```python
from build123d import *

# Parameters (mm, degrees)
SKETCH1_W           = 11.8
SKETCH1_H           = 22.5
BOSS_EXTRUDE1_DEPTH = 23.3
SKETCH2_W           = 11.8
SKETCH2_H           = 31.9
SKETCH2_R           = 1
BOSS_EXTRUDE2_DEPTH = 2.5
SKETCH3_R           = 5.9
SKETCH3_R_2         = 2.5
BOSS_EXTRUDE3_DEPTH = 4
SKETCH4_R           = 2.3
BOSS_EXTRUDE4_DEPTH = 3.2
SKETCH5_W           = 3.6
SKETCH5_H           = 1.2
BOSS_EXTRUDE5_DEPTH = 8


with BuildPart() as part:
    # Sketch1 → Boss-Extrude1 (new body)
    with BuildSketch(Plane(origin=(0, 0, 0), x_dir=(1, 0, 0), z_dir=(0, 1, 0))):
        Rectangle(SKETCH1_W, SKETCH1_H)
    extrude(amount=BOSS_EXTRUDE1_DEPTH)

    # Sketch2 → Boss-Extrude2 (add)
    with BuildSketch(Plane(origin=(0, 16.6, 0), x_dir=(1, 0, 0), z_dir=(0, 1, 0))):
        Rectangle(SKETCH2_W, SKETCH2_H)
        with Locations(Location((0, 13.65, 0), (0, 0, 270))):
            Circle(SKETCH2_R, mode=Mode.SUBTRACT)
        with Locations(Location((0, -13.65, 0), (0, 0, 90))):
            Circle(SKETCH2_R, mode=Mode.SUBTRACT)
    extrude(amount=BOSS_EXTRUDE2_DEPTH)

    # Sketch3 → Boss-Extrude3 (add)
    with BuildSketch(Plane(origin=(0, 23.3, 0), x_dir=(1, 0, 0), z_dir=(0, 1, 0))):
        with Locations((0, -5.35)):
            Circle(SKETCH3_R)
        with Locations((0, 0.95)):
            Circle(SKETCH3_R_2)
    extrude(amount=BOSS_EXTRUDE3_DEPTH)

    # Sketch4 → Boss-Extrude4 (add)
    with BuildSketch(Plane(origin=(0, 27.3, 0), x_dir=(1, 0, 0), z_dir=(0, 1, 0))):
        with Locations(Location((0, -5.35, 0), (0, 0, 270))):
            Circle(SKETCH4_R)
    extrude(amount=BOSS_EXTRUDE4_DEPTH)

    # Sketch5 → Boss-Extrude5 (add)
    with BuildSketch(Plane.XY.offset(11.25)):
        with Locations((0, 5.1)):
            Rectangle(SKETCH5_W, SKETCH5_H)
    extrude(amount=BOSS_EXTRUDE5_DEPTH)


solid = part.part
```
Check sheet for the modelled part. Datum: model origin and axes. Units: mm. A direction names the side the tool comes from. Round coordinates to 2 decimals unless told otherwise and drop trailing zeros. Loops run counter-clockwise (first coordinate to the right, second up) from the corner with the lowest first, then second, coordinate; pieces in that order, holes last. Notation, with made-up numbers: (70.5, 9) -> (99.5, 9) arc R32 cw to (99.5, 47) -> close; hole circle Ø4 at (76, 85). An arc over 180 degrees is marked (long way). Write item = value, one per line. Start each with the question number.
1) Release check for a two-part mould opening along X. For faces 1 (the flat face through (0, 0, 0)), 2 (the flat face through (-5.9, 11, 0)), 3 (the cylindrical face through (-0.226, 25.272, 11.246)), 4 (the cylindrical face through (-0.383, 17.833, -12.726)) record: released by +X, released by -X, zero draft, split by the parting line, or undercut.
2) Gauge pin test, flat ends, axial feed: pin 1 Ø4 at (x, z) = (1.5, 11.5) entering from +Y; pin 2 Ø1.3 at (x, y) = (2, 21) entering from +Z; pin 3 Ø1.4 at (x, z) = (3, -13.5) entering from -Y. Record the tip position at first contact, or that the pin passes through.
3) Set-up check for faces 5 (the flat face through (0, 18, 15.95)), 6 (the cylindrical face through (0.691, 28.878, 7.544)), 7 (the flat face through (-5, 23.3, 10)), 8 (the flat face through (0, 16.6, -15)): record each of +Z, -Z, +X, -X, +Y, -Y from which the full face is reachable in a straight line by a thin tool's end or side.
4) Sectioned sample at B-B, the plane z = -0.95. Record the cut outline in (x, y).
5) Sectioned sample at A-A, the plane z = 13.65. Record the cut outline in (x, y).
6) Thickness scan on probe 1 along Y at (x, z) = (-5, 3); probe 2 along X at (y, z) = (17.1, -13.65); probe 3 along Z at (x, y) = (-5, 21.5). Record the ranges inside material, lowest first.
7) Sectioned sample at D-D, the plane x = 3.75. Record the cut outline in (y, z), plus the area to 3 significant figures.
8) Sectioned sample at C-C, the plane y = 12. Record the cut outline in (x, z).
Results are:
q1.face_1 = zero draft
q1.face_2 = released by -X
q1.face_3 = split by the parting line
q1.face_4 = undercut
q2.pin_1 = 27.3
q2.pin_2 = 11.25
q2.pin_3 = 16.6
q3.face_5 = +Z, +X, -X, +Y
q3.face_6 = +Y
q3.face_7 = +Z, -X, +Y
q3.face_8 = -Z, +X, -X, -Y
q4.outline = (-5.9, 0) -> (5.9, 0) -> (5.9, 23.3) -> (2.5, 23.3) -> (2.5, 27.3) -> (-2.5, 27.3) -> (-2.5, 23.3) -> (-5.9, 23.3) -> close
q5.outline = (-5.9, 16.6) -> (-1, 16.6) -> (-1, 19.1) -> (-5.9, 19.1) -> close; (-1.8, 4.5) -> (1.8, 4.5) -> (1.8, 5.7) -> (-1.8, 5.7) -> close; (1, 16.6) -> (5.9, 16.6) -> (5.9, 19.1) -> (1, 19.1) -> close
q6.probe_1 = 0 to 27.3
q6.probe_2 = -5.9 to -1, 1 to 5.9
q6.probe_3 = -11.25 to 11.25
q7.outline = (0, -11.25) -> (16.6, -11.25) -> (16.6, -15.95) -> (19.1, -15.95) -> (19.1, -11.25) -> (23.3, -11.25) -> (23.3, 0.8) -> (27.3, 0.8) -> (27.3, 9.9) -> (23.3, 9.9) -> (23.3, 11.25) -> (19.1, 11.25) -> (19.1, 15.95) -> (16.6, 15.95) -> (16.6, 11.25) -> (0, 11.25) -> close
q7.area = 584 mm^2
q8.outline = (-5.9, -11.25) -> (5.9, -11.25) -> (5.9, 11.25) -> (-5.9, 11.25) -> close
